Work out the finished part from the listing and answer in its coordinate system (mm). Round coordinates to 2 decimals unless told otherwise and drop trailing zeros. Write each loop counter-clockwise with the first axis right and the second up, starting at its lowest first coordinate (ties: lowest second). Pieces come first, ordered by that corner, then holes. Notation, with made-up numbers: (36.25, -6) - (59.25, -6) arc R23 ccw to (59.25, 15) - close; hole circle Ø7 at (50.5, 58). An arc over 180 degrees is marked (long way). Write item = value, one per line. Start each with the question number.
from build123d import *

# Parameters (mm, degrees)
F0_W     = 50.8
F0_H     = 381
F0_R     = 6.35
F1_DEPTH = 1.7145
F2_SIZE  = 2.54
F3_SIZE  = 0.7874


with BuildPart() as f1:
    # F0 (on Top) → F1 (new body, symmetric)
    with BuildSketch(Plane.XY):
        Rectangle(F0_W, F0_H)
        with Locations((0, -165.1)):
            Circle(F0_R, mode=Mode.SUBTRACT)
        with Locations((0, 165.1)):
            Circle(F0_R, mode=Mode.SUBTRACT)
    extrude(amount=F1_DEPTH, both=True)

    # F2
    f2_edges = [f1.edges().sort_by_distance(p)[0] for p in [
        (25.4, -190.5, 0),
        (-25.4, -190.5, 0),
        (-25.4, 190.5, 0),
        (25.4, 190.5, 0),
    ]]
    chamfer(f2_edges, length=F2_SIZE)

    # F3
    f3_edges = [f1.edges().sort_by_distance(p)[0] for p in [
        (-6.35, -165.1, 1.7145),
        (-6.35, 165.1, 1.7145),
    ]]
    chamfer(f3_edges, length=F3_SIZE)


solid = f1.part
1. Find section B-B on x = 0. Give the vertices of the cut face in (y, z), plus the area to 3 significant figures.
2. For a pull along X with two mould halves and no side action, classify faces 1 (the face through (0, 3, -1.714)), 2 (the face through (-1.38, 158.9, -0.41)) as released by +X, released by -X, zero draft, split by the parting line, or undercut.
3. Consider line 1 (Y direction, x = 0, z = -0.5); line 2 (Y direction, x = 3.5, z = -1.15); line 3 (X direction, y = 168, z = 0.9). Determine where each line is inside the solid, lowest interval first.
4. Find section A-A on y = 165.1. Give the vertices of the cut face in (x, z).
Answer key:
q1.outline = (-190.5, -1.71) - (-171.45, -1.71) - (-171.45, 0.93) - (-172.24, 1.71) - (-190.5, 1.71) - close; (-158.75, -1.71) - (158.75, -1.71) - (158.75, 0.93) - (157.96, 1.71) - (-157.96, 1.71) - (-158.75, 0.93) - close; (171.45, -1.71) - (190.5, -1.71) - (190.5, 1.71) - (172.24, 1.71) - (171.45, 0.93) - close
q1.area = 1,220 mm²
q2.face_1 = zero draft
q2.face_2 = undercut
q3.line_1 = -190.5 to -171.45, -158.75 to 158.75, 171.45 to 190.5
q3.line_2 = -190.5 to -170.4, -159.8 to 159.8, 170.4 to 190.5
q3.line_3 = -25.4 to -5.65, 5.65 to 25.4
q4.outline = (-25.4, -1.71) - (-6.35, -1.71) - (-6.35, 0.93) - (-7.14, 1.71) - (-25.4, 1.71) - close; (6.35, -1.71) - (25.4, -1.71) - (25.4, 1.71) - (7.14, 1.71) - (6.35, 0.93) - close
